CAD build for the part. Positions are in the model's coordinates, mm. A direction names the side the tool comes from. Coordinates: 2 decimals unless noted, no trailing zeros. Loops run counter-clockwise (first coordinate to the right, second up) from the corner with the lowest first, then second, coordinate; pieces in that order, holes last. Notation, with made-up numbers: (82.5, 20) -> (107.5, 20) arc R18 ccw to (107.5, 37) -> close; hole circle Ø6 at (1.25, 86.5). An arc over 180 degrees is marked (long way). Answer as CSV lines item,"result". Start each with the question number.
```python
from build123d import *

# Parameters (mm, degrees)
SKETCH_1_R      = 1.6
SKETCH_1_R_2    = 5
EXTRUDE_1_DEPTH = 1.5


with BuildPart() as part:
    # Эскиз1 → Бобышка-Вытянуть1 (new, symmetric)
    with BuildSketch(Plane.XY):
        with BuildLine():
            Line((-22, 4), (-15.556349186, 4))
            ThreePointArc((-15.556349186, 4), (-7.384776311, 7.384776311), (-4, 15.556349186))
            Line((-4, 15.556349186), (-4, 22))
            ThreePointArc((-4, 22), (0, 26), (4, 22))
            Line((4, 22), (4, 15.556349186))
            ThreePointArc((4, 15.556349186), (7.384776311, 7.384776311), (15.556349186, 4))
            Line((15.556349186, 4), (22, 4))
            ThreePointArc((22, 4), (26, 0), (22, -4))
            Line((22, -4), (15.556349186, -4))
            ThreePointArc((15.556349186, -4), (7.384776311, -7.384776311), (4, -15.556349186))
            Line((4, -15.556349186), (4, -22))
            ThreePointArc((4, -22), (0, -26), (-4, -22))
            Line((-4, -22), (-4, -15.556349186))
            ThreePointArc((-4, -15.556349186), (-7.384776311, -7.384776311), (-15.556349186, -4))
            Line((-15.556349186, -4), (-22, -4))
            ThreePointArc((-22, -4), (-26, 0), (-22, 4))
        make_face()
        with Locations((0, 22)):
            Circle(SKETCH_1_R, mode=Mode.SUBTRACT)
        with Locations((22, 0)):
            Circle(SKETCH_1_R, mode=Mode.SUBTRACT)
        with Locations((0, -22)):
            Circle(SKETCH_1_R, mode=Mode.SUBTRACT)
        with Locations((-22, 0)):
            Circle(SKETCH_1_R, mode=Mode.SUBTRACT)
        Circle(SKETCH_1_R_2, mode=Mode.SUBTRACT)
        with Locations((-9.5, 0)):
            Circle(SKETCH_1_R, mode=Mode.SUBTRACT)
        with Locations((9.5, 0)):
            Circle(SKETCH_1_R, mode=Mode.SUBTRACT)
        with Locations((0, 12.5)):
            Circle(SKETCH_1_R, mode=Mode.SUBTRACT)
        with Locations((0, -12.5)):
            Circle(SKETCH_1_R, mode=Mode.SUBTRACT)
    extrude(amount=EXTRUDE_1_DEPTH, both=True)


solid = part.part
```
Q1. Which spindle directions (+Z, -Z, +X, -X, +Y, -Y) get a long thin tool onto all of the face, cutting with end or side? Do faces 4 (the flat face through (19, 4, 0)), 5 (the flat face through (4, -19, 0)), 6 (the flat face through (-19, -4, 0)). Say none if no direction does.
Q2. Saw through at C-C (x = -7). List the corners of the cut face in (y, z).
Q3. Saw through at D-D (y = 12.5). List the corners of the cut face in (x, z), and give its area (3 significant figures).
Q4. Pin check, flat tips, straight feed: pin 1 Ø5 at (x, y) = (0, 22) entering from +Z; pin 2 Ø0.9 at (x, z) = (20, -0.5) entering from -Y; pin 3 Ø0.9 at (x, z) = (-19.5, 0) entering from +Y; pin 4 Ø1.9 at (x, y) = (0, -12.5) entering from -Z. Stop position of each tip, or through.
Q5. Probe probe 1 along Y at (x, z) = (0, -0.8); probe 2 along Y at (x, z) = (0.5, -0.3); probe 3 along Y at (x, z) = (-22, -0.25). List the from-to ranges inside material, lowest first. Write a range as from..to.
Q6. Saw through at B-B (y = 3). List the corners of the cut face in (x, z).
Q7. Saw through at A-A (z = 0.2). Give the number of separate pieces and of enclosed holes in the cut face, and give its area (3 significant figures).
Q8. Two-plate mould, pull along X, no slides. Class faces 1 (the cylindrical face through (-1.08, -4.88, -0.02)), 2 (the cylindrical face through (-7.295, -7.475, 0.021)), 3 (the flat face through (-19, 4, 0)): pulls with the +X half, pulls with the -X half, needs draft (parallel to the pull), parting line crosses it, or undercut.
Ans:
1,face 4,"+Z, -Z, +X, +Y"
1,face 5,"+Z, -Z, +X, -Y"
1,face 6,"+Z, -Z, -X, -Y"
2,outline,"(-7.79, -1.5) -> (7.79, -1.5) -> (7.79, 1.5) -> (-7.79, 1.5) -> close"
3,outline,"(-4.41, -1.5) -> (-1.6, -1.5) -> (-1.6, 1.5) -> (-4.41, 1.5) -> close; (1.6, -1.5) -> (4.41, -1.5) -> (4.41, 1.5) -> (1.6, 1.5) -> close"
3,area,"16.9 mm²"
4,pin 1,"stops at z = 1.5"
4,pin 2,"stops at y = -4"
4,pin 3,"stops at y = 4"
4,pin 4,"passes through"
5,probe 1,"y = -26..-23.6, -20.4..-14.1, -10.9..-5, 5..10.9, 14.1..20.4, 23.6..26"
5,probe 2,"y = -25.97..-23.52, -20.48..-14.02, -10.98..-4.97, 4.97..10.98, 14.02..20.48, 23.52..25.97"
5,probe 3,"y = -4..-1.6, 1.6..4"
6,outline,"(-24.65, -1.5) -> (-4, -1.5) -> (-4, 1.5) -> (-24.65, 1.5) -> close; (4, -1.5) -> (24.65, -1.5) -> (24.65, 1.5) -> (4, 1.5) -> close"
7,separate pieces,"1"
7,enclosed holes,"9"
7,area,"712 mm²"
8,face 1,"undercut"
8,face 2,"pulls with the -X half"
8,face 3,"needs draft"
